Check sheet for the modelled part. Datum: model origin and axes. Units: mm. Round coordinates to 2 decimals unless told otherwise and drop trailing zeros.
Q1. Scan lines: probe 1 along Y at (x, z) = (24, 4.5); probe 2 along Y at (x, z) = (-3.5, 4.75); probe 3 along X at (y, z) = (214.75, 3). Record each from-to range of solid material in increasing order.
Q2. Depth check by flat-ended pin: P1, Ø4.5, axis at x = 252.62, y = 229.92, coming from the +Z side; P2, Ø3, axis at x = -29.38, y = 229.92, coming from the +Z side. Enter the tip coordinate at first touch or a pass-through.
Q3. Cross-section at A-A on z = 4. Give the number of separate pieces and of enclosed holes in the cut face, then the cut area to 3 significant figures.
from build123d import *

# Parameters (mm, degrees)
SKETCH1_W           = 304.8
SKETCH1_H           = 25
BOSS_EXTRUDE1_DEPTH = 6.35
SKETCH2_R           = 1.7
CUT_EXTRUDE1_DEPTH  = 10
SKETCH3_R           = 1.7
CUT_EXTRUDE2_DEPTH  = 22


with BuildPart() as part:
    # Sketch1 → Boss-Extrude1 (new body)
    with BuildSketch(Plane.XY):
        with Locations((111.623766163, 223.42362241)):
            Rectangle(SKETCH1_W, SKETCH1_H)
    extrude(amount=BOSS_EXTRUDE1_DEPTH)

    # Sketch2 → Cut-Extrude1 (cut)
    with BuildSketch(Plane.XY.offset(6.35)):
        with Locations((225.573766163, 216.92362241)):
            Circle(SKETCH2_R)
        with Locations((225.573766163, 229.92362241)):
            Circle(SKETCH2_R)
        with Locations((252.623766163, 229.92362241)):
            Circle(SKETCH2_R)
        with Locations((252.623766163, 216.92362241)):
            Circle(SKETCH2_R)
        with Locations((-2.326233837, 216.92362241)):
            Circle(SKETCH2_R)
        with Locations((-29.376233837, 216.92362241)):
            Circle(SKETCH2_R)
        with Locations((-29.376233837, 229.92362241)):
            Circle(SKETCH2_R)
        with Locations((-2.326233837, 229.92362241)):
            Circle(SKETCH2_R)
    extrude(amount=-CUT_EXTRUDE1_DEPTH, mode=Mode.SUBTRACT)

    # Sketch3 → Cut-Extrude2 (cut)
    with BuildSketch(Plane.XY.offset(6.35)):
        with Locations((225.573766163, 216.92362241)):
            Circle(SKETCH3_R)
        with Locations((225.573766163, 229.92362241)):
            Circle(SKETCH3_R)
        with Locations((199.050473293, 216.92362241)):
            Circle(SKETCH3_R)
        with Locations((199.050473293, 229.92362241)):
            Circle(SKETCH3_R)
        with Locations((129.123766163, 215.92362241)):
            Circle(SKETCH3_R)
        with Locations((129.123766163, 230.92362241)):
            Circle(SKETCH3_R)
        with Locations((93.960167873, 215.92362241)):
            Circle(SKETCH3_R)
        with Locations((93.960167873, 230.92362241)):
            Circle(SKETCH3_R)
        with Locations((24.196928947, 229.840552731)):
            Circle(SKETCH3_R)
        with Locations((24.156213572, 216.84061649)):
            Circle(SKETCH3_R)
    extrude(amount=-CUT_EXTRUDE2_DEPTH, mode=Mode.SUBTRACT)


solid = part.part
Results found:
1. probe 1: y = 210.92 to 215.15, 218.53 to 228.15, 231.53 to 235.92
1. probe 2: y = 210.92 to 215.69, 218.15 to 228.69, 231.15 to 235.92
1. probe 3: x = -40.78 to 92.73, 95.19 to 127.89, 130.35 to 264.02
2. P1: stops at z = 6.35
2. P2: passes through
3. separate pieces: 1
3. enclosed holes: 16
3. area: 7,470 mm2
